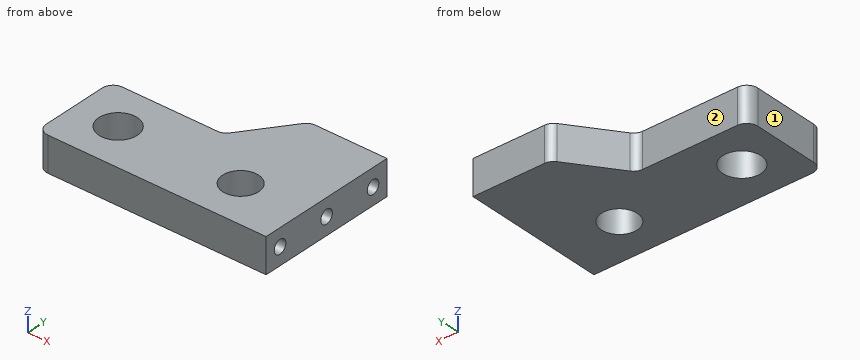
from build123d import *

# Parameters (mm, degrees)
SKETCH1_W           = 41.782
SKETCH1_H           = 16
BOSS_EXTRUDE1_DEPTH = 6.35
SKETCH1_6_R         = 3.275
CUT_EXTRUDE1_DEPTH  = 6.35
FILLET1_R           = 2
SKETCH2_R           = 1.25
CUT_EXTRUDE2_DEPTH  = 4
BOSS_EXTRUDE2_DEPTH = 6.35
FILLET2_R           = 2
SKETCH4_R           = 1.25
CUT_EXTRUDE3_DEPTH  = 4


with BuildPart() as part:
    # Sketch1 → Boss-Extrude1 (new body)
    with BuildSketch(Plane.XY):
        with Locations((20.891, 8)):
            Rectangle(SKETCH1_W, SKETCH1_H)
    extrude(amount=BOSS_EXTRUDE1_DEPTH)

    # Sketch1_6 → Cut-Extrude1 (cut)
    with BuildSketch(Plane.XY):
        with BuildLine():
            ThreePointArc((4.5, 8), (8, 4.5), (11.5, 8))
            Line((11.5, 8), (4.5, 8))
        make_face()
        with BuildLine():
            Line((4.5, 8), (11.5, 8))
            ThreePointArc((11.5, 8), (8, 11.5), (4.5, 8))
        make_face()
        with Locations((30.352, 8)):
            Circle(SKETCH1_6_R)
    extrude(amount=CUT_EXTRUDE1_DEPTH, mode=Mode.SUBTRACT)

    # Fillet1
    fillet1_edges = [part.edges().sort_by_distance(p)[0] for p in [
        (0, 0, 3.175),
        (0, 16, 3.175),
    ]]
    fillet(fillet1_edges, radius=FILLET1_R)

    # Sketch2 → Cut-Extrude2 (cut)
    with BuildSketch(Plane(origin=(41.782, 0, 0), x_dir=(0, 0, -1), z_dir=(1, 0, 0))):
        with Locations((-3.175, 13)):
            Circle(SKETCH2_R)
        with Locations((-3.175, 3)):
            Circle(SKETCH2_R)
    extrude(amount=-CUT_EXTRUDE2_DEPTH, mode=Mode.SUBTRACT)

    # Sketch3 → Boss-Extrude2 (add)
    with BuildSketch(Plane.XY.offset(6.35)):
        Polygon((20.326281713, 16), (41.782, 16), (41.782, 26), (27.712043107, 26), align=None)
    extrude(amount=-BOSS_EXTRUDE2_DEPTH)

    # Fillet2
    fillet2_edges = [part.edges().sort_by_distance(p)[0] for p in [
        (20.326281713, 16, 3.175),
        (27.712043107, 26, 3.175),
    ]]
    fillet(fillet2_edges, radius=FILLET2_R)

    # Sketch4 → Cut-Extrude3 (cut)
    with BuildSketch(Plane(origin=(41.782, 0, 0), x_dir=(0, 0, -1), z_dir=(1, 0, 0))):
        with Locations((-3.10572404, 23)):
            Circle(SKETCH4_R)
    extrude(amount=-CUT_EXTRUDE3_DEPTH, mode=Mode.SUBTRACT)


solid = part.part
Could you check a few things on this model? Use its own coordinates, in mm. Face numbers are marked on the shaded views. A direction names the side the tool comes from. Coordinates: 2 decimals unless noted, no trailing zeros. Order: outer loops, then holes, each group sorted by start corner. A loop starts at its lowest first (then second) coordinate and runs counter-clockwise, first axis right, second up.
Q1. Suppose I cut it at A-A on z = 1.25. Please give me the cut outline in (x, y) (3 decimals), and give its area (3 significant figures).
Q2. Please list where these lines run through material, in increasing order: L1, parallel to Y at x = 19, z = 0.5; L2, parallel to X at y = 6.25, z = 4.5; L3, parallel to Y at x = 11, z = 2.
Q3. Suppose I cut it at B-B on y = 3. Please give me the cut outline in (x, z) (3 decimals), and give its area (3 significant figures).
Q4. Which directions (+Z, -Z, +X, -X, +Y, -Y) give clear straight access to the entire face, cutting with the end or side of a thin tool? Please do the marked faces 1 and 2.
Q5. Suppose I cut it at D-D on y = 9.75. Please give me the cut outline in (x, z).
Q6. Will these pins go through, and if not, where does the flat tip stop? pin 1 (1 mm diameter, centred on x = 19.5, z = 4, fed in from +Y); pin 2 (5.5 mm diameter, centred on x = 8, y = 8, fed in from -Z) (3 decimals); pin 3 (1.5 mm diameter, centred on y = 13, z = 3.175, fed in from +X); pin 4 (3 mm diameter, centred on x = 14, z = 4, fed in from +Y).
Q7. Suppose I cut it at C-C on x = 28. Please give me the cut outline in (y, z).
Answer:
1. outline: (0, 2) arc R2 ccw to (2, 0) - (41.782, 0) - (41.782, 26) - (28.721, 26) arc R2 ccw to (27.112, 25.188) - (20.926, 16.812) arc R2 cw to (19.317, 16) - (2, 16) arc R2 ccw to (0, 14) - close; hole circle Ø7 at (8, 8); hole circle Ø6.55 at (30.352, 8)
1. area: 772 mm2
2. L1: y = 0 to 16
2. L2: x = 0 to 4.97, 11.03 to 27.58, 33.12 to 41.78
2. L3: y = 0 to 6.2, 9.8 to 16
3. outline: (0, 0) - (41.782, 0) - (41.782, 1.925) - (37.782, 1.925) - (37.782, 4.425) - (41.782, 4.425) - (41.782, 6.35) - (0, 6.35) - close
3. area: 255 mm2
4. face 1: +Z, -Z, -X, +Y, -Y
4. face 2: +Z, -Z, -X, +Y
5. outline: (0, 0) - (4.97, 0) - (4.97, 6.35) - (0, 6.35) - close; (11.03, 0) - (27.58, 0) - (27.58, 6.35) - (11.03, 6.35) - close; (33.12, 0) - (41.78, 0) - (41.78, 6.35) - (33.12, 6.35) - close
6. pin 1: stops at y = 16.12
6. pin 2: passes through
6. pin 3: stops at x = 37.78
6. pin 4: stops at y = 16
7. outline: (0, 0) - (5.72, 0) - (5.72, 6.35) - (0, 6.35) - close; (10.28, 0) - (25.87, 0) - (25.87, 6.35) - (10.28, 6.35) - close
